Part model, mm, in its own coordinate system. A direction names the side the tool comes from. Round coordinates to 2 decimals unless told otherwise and drop trailing zeros. Write each loop counter-clockwise with the first axis right and the second up, starting at its lowest first coordinate (ties: lowest second). Pieces come first, ordered by that corner, then holes. Notation, with made-up numbers: M 48.25,82 L 104.25,82 A9 ccw 104.25,86 Z; hole C -10.5,-4.5 d7. An arc over 180 degrees is marked long. Use one line per item in the form item = value. Start each with the question number.
Item 1: Cut at D-D, the plane y = 46. Give the cut face in (x, z).
Item 2: Flat gauge pins, fed straight in: pin 1 Ø17 at (x, y) = (84, 34.5) entering from +Z; pin 2 Ø10.5 at (x, z) = (174, 14.5) entering from +Y; pin 3 Ø4 at (y, z) = (71.5, 27.5) entering from +X. Where does each tip first touch, or does it go through?
Item 3: Which spindle directions (+Z, -Z, +X, -X, +Y, -Y) get a long thin tool onto all of the face, cutting with end or side? Do faces 4 (the face through (67.5, 28, 20)), 5 (the face through (95, 115, 15)), 6 (the face through (29, 57.5, 20)), 7 (the face through (164, 57.5, 20)). Say none if no direction does.
Item 4: Cut at B-B, the plane x = 47. Give the cut face in (y, z).
Item 5: Cut at C-C, the plane z = 20. Give the cut face in (x, y), then the cut area to 3 significant figures.
Item 6: Probe L1, parallel to X at y = 50.5, z = 8.5; L2, parallel to X at y = 61, z = 22.5; L3, parallel to Y at x = 138, z = 31. List the from-to ranges inside material, lowest first.
Item 7: Mould opens along X. For faces 1 (the face through (0, 33, 19)), 2 (the face through (95, 58, 38)), 3 (the face through (125, 29, 20)) say: +X half, -X half, draft (parallel to the pull), parting line (faces both ways), or undercut.
Item 8: Cut at A-A, the plane y = 100. Give the cut face in (x, z), then the cut area to 3 significant figures.
from build123d import *

# Parameters (mm, degrees)
SKETCH1_W           = 192.5
SKETCH1_H           = 115
BOSS_EXTRUDE1_DEPTH = 3
BOSS_EXTRUDE2_DEPTH = 35


with BuildPart() as part:
    # Sketch1 → Boss-Extrude1 (new body)
    with BuildSketch(Plane.XY):
        with Locations((96.25, 57.5)):
            Rectangle(SKETCH1_W, SKETCH1_H)
    extrude(amount=BOSS_EXTRUDE1_DEPTH)

    # Sketch2 → Boss-Extrude2 (add)
    with BuildSketch(Plane.XY.offset(3)):
        Polygon((0, 57.5), (0, 0), (67.5, 0), (67.5, 57.5), (125, 57.5), (125, 0), (192.5, 0), (192.5, 57.5), (135, 57.5), (135, 115), (57.5, 115), (57.5, 57.5), align=None)
    extrude(amount=BOSS_EXTRUDE2_DEPTH)


solid = part.part
Model answer:
q1.outline = M 0,0 L 192.5,0 L 192.5,38 L 125,38 L 125,3 L 67.5,3 L 67.5,38 L 0,38 Z
q2.pin_1 = 3
q2.pin_2 = 57.5
q2.pin_3 = 135
q3.face_4 = +Z, -Y
q3.face_5 = +Z, -Z, +X, -X, +Y
q3.face_6 = +Z, -X, +Y
q3.face_7 = +Z, +X, +Y
q4.outline = M 0,0 L 115,0 L 115,3 L 57.5,3 L 57.5,38 L 0,38 Z
q5.outline = M 0,0 L 67.5,0 L 67.5,57.5 L 125,57.5 L 125,0 L 192.5,0 L 192.5,57.5 L 135,57.5 L 135,115 L 57.5,115 L 57.5,57.5 L 0,57.5 Z
q5.area = 12,200 mm²
q6.L1 = 0 to 67.5, 125 to 192.5
q6.L2 = 57.5 to 135
q6.L3 = 0 to 57.5
q7.face_1 = -X half
q7.face_2 = draft
q7.face_3 = undercut
q8.outline = M 0,0 L 192.5,0 L 192.5,3 L 135,3 L 135,38 L 57.5,38 L 57.5,3 L 0,3 Z
q8.area = 3,290 mm²
